Source: CAD feature listing. Evaluate the final solid. Frame: model axes, mm. A direction names the side the tool comes from. Give positions to 0.01 mm unless a question says otherwise; leave off trailing zeros. Order: outer loops, then holes, each group sorted by start corner. A loop starts at its lowest first (then second) coordinate and runs counter-clockwise, first axis right, second up. Notation, with made-up numbers: (64.25, -8) -> (98.25, -8) arc R23 ccw to (98.25, 31) -> close; hole circle Ø10 at (29.5, 43). An arc over 180 degrees is marked (long way). Answer in a Markdown table with one row per item.
Autodesk Inventor part; units mm, degrees
ref_plane "YZ Plane" through (0, 0, 0) normal (1, 0, 0) x (0, 1, 0)
ref_plane "XY Plane" through (0, 0, 0) normal (0, 0, 1) x (1, 0, 0)
sketch "Sketch1" plane through (0, 0, 0) normal (0, 0, 1) x (1, 0, 0)
  circle A0 centre (0, 0) radius 5
  dimension "d0" = 10
extrude "Extrusion1" add sketch "Sketch1" along normal blind 10
sketch "Sketch2" plane through (0, 0, 10) normal (0, 0, 1) x (1, 0, 0)
  circle A0 centre (0, 0) radius 5
  circle A1 centre (0, 0) radius 0.8
  dimension "d3" = 1.6
extrude "Extrusion2" cut sketch "Sketch2" against normal blind 2 contours A1
sketch "Sketch3" plane through (0, 0, 10) normal (0, 0, 1) x (1, 0, 0)
  circle A0 centre (0, 0) radius 0.8
  circle A1 centre (0, 0) radius 5
ref_plane "Work Plane1" through (0, 5, 0) normal (0, 1, 0) x (-1, 0, 0)
sketch "Sketch4" plane through (0, 5, 0) normal (0, 1, 0) x (-1, 0, 0)
  line L0 (-5, 0) -> (-5, 10)
  line L1 (5, 0) -> (5, 10)
  line L2 (0, -2) -> (0, 12)
  line L3 (-5, 10) -> (5, 10)
  point P0 (0, 0)
  point P1 (0, 9)
  dimension "d8" = 1
hole "Hole1" at (0, 5, 9) direction (0, -1, 0) diameter 1.181 depth 5
sketch "Sketch5" plane through (0, 0, 10) normal (0, 0, 1) x (1, 0, 0)
  circle A0 centre (0, 0) radius 5
  circle A1 centre (0, 0) radius 2.5
  circle A2 centre (0, 0) radius 5
  dimension "d16" = 5
extrude "Extrusion3" cut sketch "Sketch5" against normal blind 4
sketch "Sketch6" plane through (0, 0, 10) normal (0, 0, 1) x (1, 0, 0)
  circle A0 centre (0, 0) radius 2.5
  circle A1 centre (0, 0) radius 0.8
sketch "Sketch7" plane through (0, 0, 6) normal (0, 0, 1) x (1, 0, 0)
  circle A0 centre (0, 0) radius 2.5
  circle A1 centre (0, -3.5) radius 0.75
  dimension "d19" = 1.5
  dimension "d20" = 3.5
extrude "Extrusion4" cut sketch "Sketch7" against normal through all contours A1
properties part number "Jig_Bearing_Asm_Housing_Holder"
(1) Section query D-D (y = 0). Return the cut outline in (x, z), plus the area to 3 significant figures.
A:
| item | result |
|---|---|
| outline | (-5, 0) -> (5, 0) -> (5, 6) -> (2.5, 6) -> (2.5, 10) -> (0.8, 10) -> (0.8, 8) -> (-0.8, 8) -> (-0.8, 10) -> (-2.5, 10) -> (-2.5, 6) -> (-5, 6) -> close |
| area | 76.8 mm^2 |
(2) Access query for faces 1 (the flat face through (2, -2, 6)), 2 (the cylindrical face through (-1.08, 4.88, 2.96)). Directions: +Z, -Z, +X, -X, +Y, -Y. A direction counts if a zero-diameter tool reaches every point of the face in a straight line with its end or side. Return the directions, or none.
A:
| item | result |
|---|---|
| face 1 | +Z |
| face 2 | +Z, -Z |
(3) Ray query, probe 1 along Y at (x, z) = (0, 1.35); probe 2 along Z at (x, y) = (1.25, -4.25); probe 3 along Z at (x, y) = (0, 1.95). Return the intervals inside material, ascending.
A:
| item | result |
|---|---|
| probe 1 | y = -5 to -4.25, -2.75 to 5 |
| probe 2 | z = 0 to 6 |
| probe 3 | z = 0 to 8.41, 9.59 to 10 |
(4) Section query C-C (z = 7.25). Return the cut outline in (x, y).
A:
| item | result |
|---|---|
| outline | circle Ø5 at (0, 0) |
(5) Section query A-A (x = -0.25). Return the cut outline in (y, z).
A:
| item | result |
|---|---|
| outline | (-4.99, 0) -> (-4.21, 0) -> (-4.21, 6) -> (-4.99, 6) -> close; (-2.79, 0) -> (4.99, 0) -> (4.99, 6) -> (2.49, 6) -> (2.49, 8.47) -> (0.76, 8.47) -> (0.76, 8) -> (-0.76, 8) -> (-0.76, 10) -> (-2.49, 10) -> (-2.49, 6) -> (-2.79, 6) -> close; (0.76, 9.53) -> (2.49, 9.53) -> (2.49, 10) -> (0.76, 10) -> close |
(6) Pull-direction query (Z, two-part tool) for faces 3 (the cylindrical face through (-0.163, -4.232, 3.042)), 4 (the cylindrical face through (-0.177, 1.506, 9.563)), 5 (the flat face through (0, 0, 0)), 6 (the flat face through (-1, 1, 10)); classes: +Z half, -Z half, draft (parallel to the pull), parting line (faces both ways), or undercut.
A:
| item | result |
|---|---|
| face 3 | draft |
| face 4 | undercut |
| face 5 | -Z half |
| face 6 | +Z half |
(7) Section query B-B (y = -3.5). Return the cut outline in (x, z).
A:
| item | result |
|---|---|
| outline | (-3.57, 0) -> (-0.75, 0) -> (-0.75, 6) -> (-3.57, 6) -> close; (0.75, 0) -> (3.57, 0) -> (3.57, 6) -> (0.75, 6) -> close |
(8) First-contact query: pin 1 Ø4 at (x, z) = (-2.5, 5) entering from -Y; pin 2 Ø4 at (x, z) = (3.5, 8.5) entering from +Y; pin 3 Ø0.8 at (x, y) = (0, 0) entering from +Z. Flat tips, straight axial feed; report the tip coordinate or a pass-through.
A:
| item | result |
|---|---|
| pin 1 | stops at y = -4.97 |
| pin 2 | stops at y = 2 |
| pin 3 | stops at z = 8 |
